Source: three-view drawing plus pictorial views. Frame: mm from the lowest corner of the part. Coordinates: 2 decimals unless noted, no trailing zeros. Write each loop counter-clockwise with the first axis right and the second up, starting at its lowest first coordinate (ties: lowest second). Pieces come first, ordered by that corner, then holes. Notation, with made-up numbers: (-30, 64.5) -> (28, 64.5) arc R18 cw to (28, 79.5) -> close; hole circle Ø4 at (33, 62). An arc over 180 degrees is marked (long way). Write item = value, one per line.
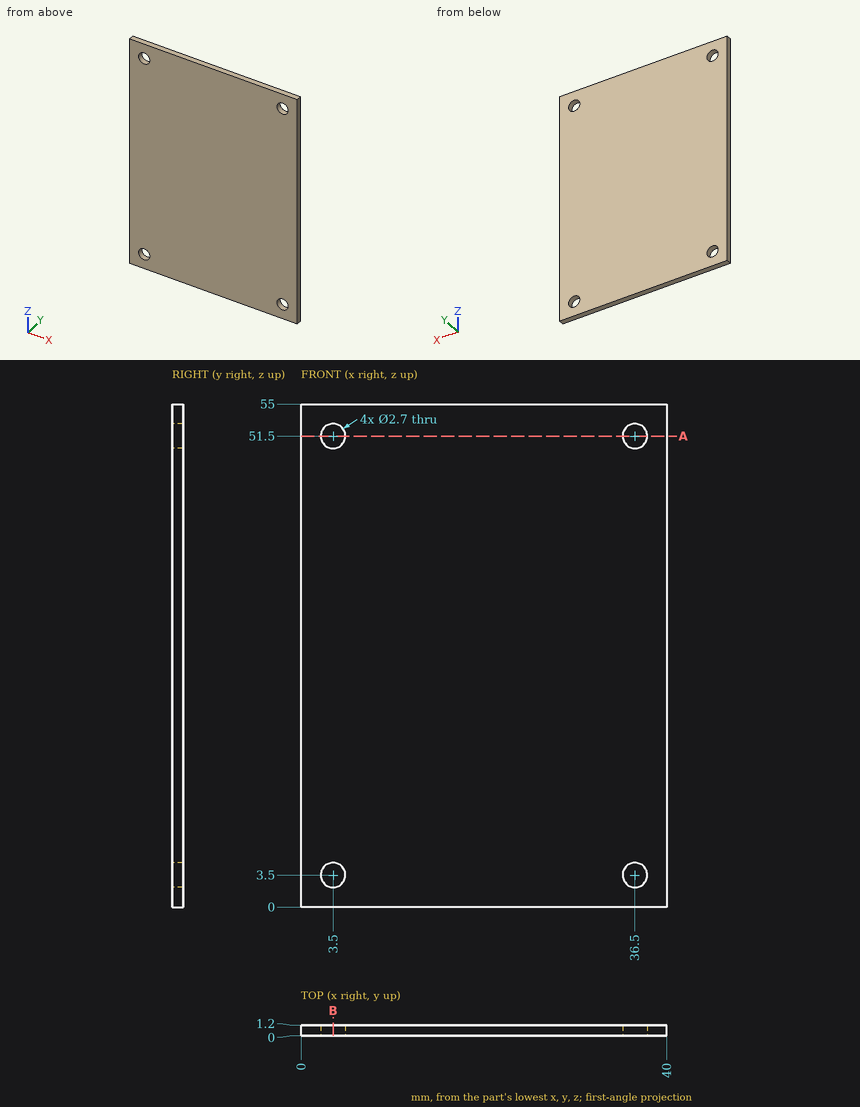
1) Material intervals for probe 1 along Z at (x, y) = (36.5, 0.85); probe 2 along X at (y, z) = (0.7, 51.5); probe 3 along X at (y, z) = (0.25, 50.5), sorted ascending. Write a range as [from, to].
Answer block:
probe_1 = [0, 2.15], [4.85, 50.15], [52.85, 55]
probe_2 = [0, 2.15], [4.85, 35.15], [37.85, 40]
probe_3 = [0, 2.59], [4.41, 35.59], [37.41, 40]
2) Cut plane B-B, the plane x = 3.5. Output: boundary loops of the cut face in (y, z).
Answer block:
outline = (0, 0) -> (1.2, 0) -> (1.2, 2.15) -> (0, 2.15) -> close; (0, 4.85) -> (1.2, 4.85) -> (1.2, 50.15) -> (0, 50.15) -> close; (0, 52.85) -> (1.2, 52.85) -> (1.2, 55) -> (0, 55) -> close
3) Cut plane A-A, the plane z = 51.5. Output: boundary loops of the cut face in (x, y), and give its area (3 significant figures).
Answer block:
outline = (0, 0) -> (2.15, 0) -> (2.15, 1.2) -> (0, 1.2) -> close; (4.85, 0) -> (35.15, 0) -> (35.15, 1.2) -> (4.85, 1.2) -> close; (37.85, 0) -> (40, 0) -> (40, 1.2) -> (37.85, 1.2) -> close
area = 41.5 mm2
